Part model, mm, in its own coordinate system. Round coordinates to 2 decimals unless told otherwise and drop trailing zeros. Put each result on its own line as item: value.
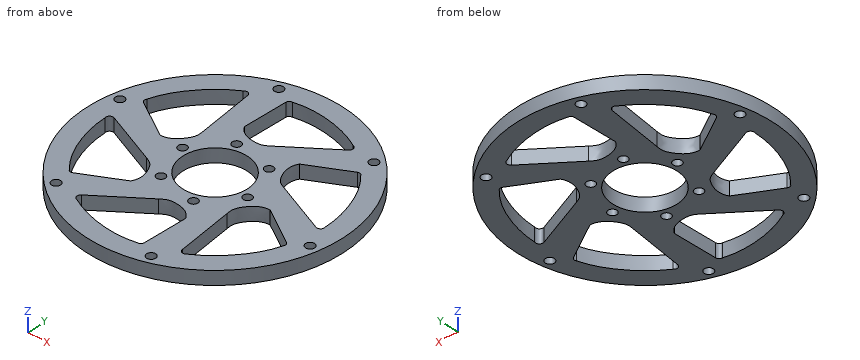
from build123d import *

# Parameters (mm, degrees)
SCHIZZO1_R                   = 37.92
SCHIZZO1_R_2                 = 1.325
SCHIZZO1_R_3                 = 9.55
SCHIZZO1_R_4                 = 1.28
ESTRUSIONE_ESTRUSIONE1_DEPTH = 4.04


with BuildPart() as part:
    # Schizzo1 → Estrusione-Estrusione1 (new body)
    with BuildSketch(Plane.XY):
        with Locations((39.644562935, 40.222708022)):
            Circle(SCHIZZO1_R)
        with Locations((28.381746106, 73.624975266)):
            Circle(SCHIZZO1_R_2, mode=Mode.SUBTRACT)
        with Locations((39.644562935, 40.222708022)):
            Circle(SCHIZZO1_R_3, mode=Mode.SUBTRACT)
        with Locations((35.774368233, 51.581475251)):
            Circle(SCHIZZO1_R_4, mode=Mode.SUBTRACT)
        with Locations((47.546446561, 49.253778566)):
            Circle(SCHIZZO1_R_4, mode=Mode.SUBTRACT)
        with Locations((62.940366498, 66.677727137)):
            Circle(SCHIZZO1_R_2, mode=Mode.SUBTRACT)
        with Locations((51.416641262, 37.895011337)):
            Circle(SCHIZZO1_R_4, mode=Mode.SUBTRACT)
        with Locations((74.203183328, 33.275459892)):
            Circle(SCHIZZO1_R_2, mode=Mode.SUBTRACT)
        with Locations((43.514757637, 28.863940793)):
            Circle(SCHIZZO1_R_4, mode=Mode.SUBTRACT)
        with Locations((50.907379765, 6.820440778)):
            Circle(SCHIZZO1_R_2, mode=Mode.SUBTRACT)
        with Locations((31.74267931, 31.191637478)):
            Circle(SCHIZZO1_R_4, mode=Mode.SUBTRACT)
        with Locations((16.348759372, 13.767688907)):
            Circle(SCHIZZO1_R_2, mode=Mode.SUBTRACT)
        with Locations((27.872484608, 42.550404707)):
            Circle(SCHIZZO1_R_4, mode=Mode.SUBTRACT)
        with Locations((5.085942543, 47.169956152)):
            Circle(SCHIZZO1_R_2, mode=Mode.SUBTRACT)
        with BuildLine():
            Line((32.537324842, 57.752341263), (32.947782143, 70.845929152))
            ThreePointArc((32.947782143, 70.845929152), (33.276613104, 71.574360929), (34.024210756, 71.856921375))
            add(Edge.make_bspline(
                [(34.024210756, 71.856921375), (37.813103061, 72.754463636), (45.237238781, 72.465064372), (52.177131888, 70.085413797), (55.180541117, 68.422554037)],
                knots=[0, 0, 0, 0, 0.531113686, 1, 1, 1, 1], degree=3))
            ThreePointArc((55.180541117, 68.422554037), (56.070695624, 67.573353666), (55.651210487, 66.416829331))
            Line((55.651210487, 66.416829331), (42.018531755, 56.173261728))
            add(Edge.make_bspline(
                [(32.537324842, 57.752341263), (33.085767208, 56.679660611), (34.829216379, 55.289156312), (37.666961886, 54.791954013), (40.192033726, 54.822389026), (41.396684563, 55.706006988), (42.018531755, 56.173261728)],
                knots=[0, 0, 0, 0, 0.332930463, 0.577052926, 0.800008074, 1, 1, 1, 1], degree=3))
        make_face(mode=Mode.SUBTRACT)
        with BuildLine():
            Line((54.645132059, 46.142067569), (70.332661194, 39.457605267))
            ThreePointArc((70.332661194, 39.457605267), (71.543983217, 39.67258265), (71.834335058, 40.868079251))
            add(Edge.make_bspline(
                [(64.230419238, 60.907182464), (66.902159789, 58.074676605), (70.363600535, 51.500486839), (71.772709238, 44.300537822), (71.834335058, 40.868079251)],
                knots=[0, 0, 0, 0, 0.531113686, 1, 1, 1, 1], degree=3))
            ThreePointArc((64.230419238, 60.907182464), (63.611915888, 61.413340799), (62.816659984, 61.333900877))
            Line((62.816659984, 61.333900877), (51.272051595, 55.142573382))
            add(Edge.make_bspline(
                [(51.272051595, 55.142573382), (50.617304082, 54.131268034), (50.284816621, 51.926144612), (51.273099553, 49.219983765), (52.561992967, 47.048424911), (53.929553988, 46.446975665), (54.645132059, 46.142067569)],
                knots=[0, 0, 0, 0, 0.332930463, 0.577052926, 0.800008074, 1, 1, 1, 1], degree=3))
        make_face(mode=Mode.SUBTRACT)
        with BuildLine():
            Line((52.271163239, 30.191513863), (54.326013642, 13.263483958))
            ThreePointArc((54.326013642, 13.263483958), (55.117850528, 12.321937006), (56.298356876, 12.668233236))
            add(Edge.make_bspline(
                [(69.850771418, 29.272969111), (68.733619663, 25.542920992), (64.770924689, 19.258130489), (59.240140286, 14.437832047), (56.298356876, 12.668233236)],
                knots=[0, 0, 0, 0, 0.531113686, 1, 1, 1, 1], degree=3))
            ThreePointArc((69.850771418, 29.272969111), (69.979865719, 30.061687892), (69.513440776, 30.710679746))
            Line((69.513440776, 30.710679746), (58.379289688, 37.61294014))
            add(Edge.make_bspline(
                [(58.379289688, 37.61294014), (57.176099809, 37.674315445), (55.100163177, 36.859696322), (53.250700602, 34.650737773), (52.014522176, 32.448743907), (52.177432361, 30.963676699), (52.271163239, 30.191513863)],
                knots=[0, 0, 0, 0, 0.332930463, 0.577052926, 0.800008074, 1, 1, 1, 1], degree=3))
        make_face(mode=Mode.SUBTRACT)
        with BuildLine():
            Line((37.270594115, 24.272154316), (23.637915383, 14.028586713))
            ThreePointArc((23.637915383, 14.028586713), (23.218430247, 12.872062378), (24.108584753, 12.022862007))
            add(Edge.make_bspline(
                [(45.264915115, 8.588494669), (41.476022809, 7.690952408), (34.051887089, 7.980351672), (27.111993983, 10.360002247), (24.108584753, 12.022862007)],
                knots=[0, 0, 0, 0, 0.531113686, 1, 1, 1, 1], degree=3))
            ThreePointArc((45.264915115, 8.588494669), (46.012512766, 8.871055115), (46.341343727, 9.599486892))
            Line((46.341343727, 9.599486892), (46.751801028, 22.693074781))
            add(Edge.make_bspline(
                [(46.751801028, 22.693074781), (46.203358662, 23.765755433), (44.459909491, 25.156259732), (41.622163984, 25.653462031), (39.097092144, 25.623027018), (37.892441308, 24.739409056), (37.270594115, 24.272154316)],
                knots=[0, 0, 0, 0, 0.332930463, 0.577052926, 0.800008074, 1, 1, 1, 1], degree=3))
        make_face(mode=Mode.SUBTRACT)
        with BuildLine():
            Line((24.643993811, 34.303348475), (8.956464676, 40.987810777))
            ThreePointArc((8.956464676, 40.987810777), (7.745142654, 40.772833394), (7.454790812, 39.577336793))
            add(Edge.make_bspline(
                [(15.058706632, 19.53823358), (12.386966081, 22.370739439), (8.925525335, 28.944929205), (7.516416632, 36.144878222), (7.454790812, 39.577336793)],
                knots=[0, 0, 0, 0, 0.531113686, 1, 1, 1, 1], degree=3))
            ThreePointArc((15.058706632, 19.53823358), (15.677209983, 19.032075245), (16.472465887, 19.111515167))
            Line((16.472465887, 19.111515167), (28.017074275, 25.302842662))
            add(Edge.make_bspline(
                [(28.017074275, 25.302842662), (28.671821788, 26.31414801), (29.004309249, 28.519271432), (28.016026317, 31.225432279), (26.727132903, 33.396991133), (25.359571882, 33.998440379), (24.643993811, 34.303348475)],
                knots=[0, 0, 0, 0, 0.332930463, 0.577052926, 0.800008074, 1, 1, 1, 1], degree=3))
        make_face(mode=Mode.SUBTRACT)
        with BuildLine():
            Line((27.017962631, 50.253902181), (24.963112228, 67.181932086))
            ThreePointArc((24.963112228, 67.181932086), (24.171275342, 68.123479038), (22.990768994, 67.777182808))
            add(Edge.make_bspline(
                [(9.438354453, 51.172446933), (10.555506207, 54.902495052), (14.518201181, 61.187285555), (20.048985584, 66.007583997), (22.990768994, 67.777182808)],
                knots=[0, 0, 0, 0, 0.531113686, 1, 1, 1, 1], degree=3))
            ThreePointArc((9.438354453, 51.172446933), (9.309260152, 50.383728152), (9.775685094, 49.734736298))
            Line((9.775685094, 49.734736298), (20.909836183, 42.832475904))
            add(Edge.make_bspline(
                [(20.909836183, 42.832475904), (22.113026061, 42.771100599), (24.188962693, 43.585719722), (26.038425268, 45.794678271), (27.274603694, 47.996672137), (27.11169351, 49.481739345), (27.017962631, 50.253902181)],
                knots=[0, 0, 0, 0, 0.332930463, 0.577052926, 0.800008074, 1, 1, 1, 1], degree=3))
        make_face(mode=Mode.SUBTRACT)
    extrude(amount=ESTRUSIONE_ESTRUSIONE1_DEPTH)


solid = part.part
1. Probe line 1 along Y through (x, z) = (36, 0.9); line 2 along X through (y, z) = (60.5, 1.2); line 3 along Y through (x, z) = (31, 0.8). List the from-to ranges inside material, lowest first. Write a range as [from, to].
A:
line 1: y = [2.48, 8.22], [23.32, 31.4], [49.05, 50.32], [52.84, 55.15], [72.23, 77.97]
line 2: x = [7.6, 14.64], [25.77, 32.62], [47.78, 61.26], [64.6, 71.69]
line 3: y = [3.3, 9.23], [19.56, 30.15], [32.23, 36.16], [44.28, 77.14]
2. Band-saw the part on A-A (x = 19). Give the number of separate pieces and of enclosed holes in the cut face, plus the area to 3 significant figures.
A:
separate pieces: 3
enclosed holes: 0
area: 107 mm²
3. Pin check, flat tip, straight feed: P1, Ø1, axis at x = 62.5, z = 0.5, coming from the -Y side. Stop position of the tip, or through.
A:
P1: stops at y = 9.59
